from build123d import *

# Parameters (mm, degrees)
RESSALTO_EXTRUS_O1_DEPTH = 10.5
RESSALTO_EXTRUS_O2_START = -0.405481833
RESSALTO_EXTRUS_O2_DEPTH = 0.405481833
ESBO_O6_R                = 1.5
ESBO_O6_R_2              = 0.439880444
ESBO_O6_R_3              = 0.420000653
CORTE_EXTRUS_O1_DEPTH    = 10
ESBO_O7_R                = 2
CORTE_EXTRUS_O2_DEPTH    = 10
ESBO_O8_W                = 16.345048289
ESBO_O8_H                = 10.10072272
CORTE_EXTRUS_O3_DEPTH    = 6


with BuildPart() as part:
    # Esboço1 → Ressalto-extrusão1 (new body)
    with BuildSketch(Plane.XZ.offset(-2000)):
        with BuildLine():
            Line((26.191736717, -104.725419486), (63.230487022, -104.725419486))
            ThreePointArc((63.230487022, -104.725419486), (64.096864483, -104.922813013), (64.79222464, -105.476029391))
            Line((64.79222464, -105.476029391), (75.753474335, -119.17759151))
            ThreePointArc((75.753474335, -119.17759151), (76.078993355, -119.764967722), (76.191736717, -120.426981605))
            Line((76.191736717, -120.426981605), (76.191736717, -135.371353563))
            ThreePointArc((76.191736717, -135.371353563), (75.847871178, -136.492611182), (74.934518069, -137.228306945))
            Line((74.934518069, -137.228306945), (56.549353262, -144.582372868))
            ThreePointArc((56.549353262, -144.582372868), (56.184786952, -144.689332259), (55.806571909, -144.725419486))
            Line((55.806571909, -144.725419486), (49.020163841, -144.725419486))
            Line((49.020163841, -144.725419486), (48.505389373, -144.65803617))
            Line((48.505389373, -144.65803617), (48.017411303, -144.455878196))
            Line((48.017411303, -144.455878196), (47.605950279, -144.139633048))
            Line((47.605950279, -144.139633048), (46.777523154, -143.311205924))
            ThreePointArc((46.777523154, -143.311205924), (46.128676457, -142.877660421), (45.363309592, -142.725419486))
            Line((45.363309592, -142.725419486), (26.191736717, -142.725419486))
            Line((26.191736717, -142.725419486), (26.191736717, -104.725419486))
        make_face()
        with BuildLine():
            Line((48.266993092, -143.386462299), (47.484629935, -142.604099142))
            ThreePointArc((47.484629935, -142.604099142), (46.511359889, -141.953780888), (45.363309592, -141.725419486))
            Line((45.363309592, -141.725419486), (27.191736717, -141.725419486))
            Line((27.191736717, -141.725419486), (27.191736717, -105.725419486))
            Line((27.191736717, -105.725419486), (63.230487022, -105.725419486))
            ThreePointArc((63.230487022, -105.725419486), (63.663675752, -105.82411625), (64.011355831, -106.100724438))
            Line((64.011355831, -106.100724438), (74.972605526, -119.802286557))
            ThreePointArc((74.972605526, -119.802286557), (75.135365036, -120.095974663), (75.191736717, -120.426981605))
            Line((75.191736717, -120.426981605), (75.191736717, -135.371353563))
            ThreePointArc((75.191736717, -135.371353563), (75.019803947, -135.931982372), (74.563127393, -136.299830254))
            Line((74.563127393, -136.299830254), (56.177962586, -143.653896177))
            ThreePointArc((56.177962586, -143.653896177), (55.995679431, -143.707375873), (55.806571909, -143.725419486))
            Line((55.806571909, -143.725419486), (49.085335215, -143.725419486))
            Line((49.085335215, -143.725419486), (48.766120713, -143.683634718))
            Line((48.766120713, -143.683634718), (48.522121146, -143.582551368))
            Line((48.522121146, -143.582551368), (48.266993092, -143.386462299))
        make_face(mode=Mode.SUBTRACT)
    extrude(amount=RESSALTO_EXTRUS_O1_DEPTH)

    # Esboço5 → Ressalto-extrusão2 (add)
    with BuildSketch(Plane.XZ.offset(-1989.5).offset(RESSALTO_EXTRUS_O2_START)):
        with BuildLine():
            Line((27.191736717, -105.725419486), (63.230487022, -105.725419486))
            ThreePointArc((63.230487022, -105.725419486), (63.663675752, -105.82411625), (64.011355831, -106.100724438))
            Line((64.011355831, -106.100724438), (74.972605526, -119.802286557))
            ThreePointArc((74.972605526, -119.802286557), (75.135365036, -120.095974663), (75.191736717, -120.426981605))
            Line((75.191736717, -120.426981605), (75.191736717, -135.371353563))
            ThreePointArc((75.191736717, -135.371353563), (75.019803947, -135.931982372), (74.563127393, -136.299830254))
            Line((74.563127393, -136.299830254), (56.177962586, -143.653896177))
            ThreePointArc((56.177962586, -143.653896177), (55.995679431, -143.707375873), (55.806571909, -143.725419486))
            Line((55.806571909, -143.725419486), (49.085335215, -143.725419486))
            ThreePointArc((49.085335215, -143.725419486), (48.642453796, -143.637327588), (48.266993092, -143.386462299))
            Line((48.266993092, -143.386462299), (47.484629935, -142.604099142))
            ThreePointArc((47.484629935, -142.604099142), (46.511359889, -141.953780888), (45.363309592, -141.725419486))
            Line((45.363309592, -141.725419486), (27.191736717, -141.725419486))
            Line((27.191736717, -141.725419486), (27.191736717, -105.725419486))
        make_face()
    extrude(amount=RESSALTO_EXTRUS_O2_DEPTH)

    # Esboço6 → Corte-extrusão1 (cut)
    with BuildSketch(Plane.XZ.offset(-1989.5)):
        with Locations(Location((51.191736717, -118.225419486, 0), (0, 0, 270))):
            Circle(ESBO_O6_R)
        with Locations(Location((51.191736717, -133.225419486, 0), (0, 0, 270))):
            Circle(ESBO_O6_R)
        with Locations(Location((72.191736717, -130.725419486, 0), (0, 0, 270))):
            Circle(ESBO_O6_R)
        with Locations(Location((53.191736717, -139.725419486, 0), (0, 0, 270))):
            Circle(ESBO_O6_R)
        with Locations(Location((28.899554792, -108.599940214, 0), (0, 0, 270))):
            Circle(ESBO_O6_R_2)
        with Locations(Location((29.339435236, -139.725419486, 0), (0, 0, 270))):
            Circle(ESBO_O6_R_3)
    extrude(amount=-CORTE_EXTRUS_O1_DEPTH, mode=Mode.SUBTRACT)

    # Esboço7 → Corte-extrusão2 (cut)
    with BuildSketch(Plane.ZY.offset(-26.191736717)):
        with Locations(Location((-137.725419486, 1995.5, 0), (0, 0, 270))):
            Circle(ESBO_O7_R)
        with Locations(Location((-109.725419486, 1995.5, 0), (0, 0, 270))):
            Circle(ESBO_O7_R)
    extrude(amount=-CORTE_EXTRUS_O2_DEPTH, mode=Mode.SUBTRACT)

    # Esboço8 → Corte-extrusão3 (cut)
    with BuildSketch(Plane(origin=(0, 0, -144.725419486), x_dir=(-1, 0, 0), z_dir=(0, 0, -1))):
        with Locations((-46.726167809, 1994.995129696)):
            Rectangle(ESBO_O8_W, ESBO_O8_H)
    extrude(amount=-CORTE_EXTRUS_O3_DEPTH, mode=Mode.SUBTRACT)


solid = part.part
Work out the finished part from the listing and answer in its coordinate system (mm). A direction names the side the tool comes from. Round coordinates to 2 decimals unless told otherwise and drop trailing zeros. Order: outer loops, then holes, each group sorted by start corner. A loop starts at its lowest first (then second) coordinate and runs counter-clockwise, first axis right, second up. Notation, with made-up numbers: M 71,45 L 95,45 A16 cw 95,51 Z; hole C 73.5,80 d11. An arc over 180 degrees is marked long. Put each result on its own line as item: value. Start each with the question number.
Q1. Section A-A, the plane y = 1995.5 is taken. Give the number of separate pieces and of enclosed holes in the cut face, and give its area (3 significant figures).
Q2. Section B-B, the plane y = 1990.75 is taken. Write down the section's boundary in (x, z), and give its area (3 significant figures).
Q3. Section C-C, the plane z = -123 is taken. Write down the section's boundary in (x, y).
Q4. Flat-ended cylindrical pins translate along their axes: pin 1 (1.1 mm diameter, centred on y = 1994.5, z = -144, fed in from -X); pin 2 (3 mm diameter, centred on x = 52.5, y = 1994, fed in from -Z); pin 3 (5 mm diameter, centred on y = 1996, z = -115.5, fed in from +X); pin 4 (6 mm diameter, centred on x = 58, y = 1996, fed in from -Z). Find the tip coordinate at first contact, or state that the pin passes through.
Q5. Section D-D, the plane x = 33 is taken. Write down the section's boundary in (y, z).
Q6. Straight lines are drawn through the part: L1, parallel to Z at x = 26.6, y = 1995.5; L2, parallel to Z at x = 35, y = 1990.5; L3, parallel to X at y = 1998.75, z = -121.5. For each, find the intervals that lie inside material, in ascending order. Write a range as [from, to].
Q7. A tool of negligible diameter and unlimited length cuts with its end or side. For faces 4 (the flat face through (34, 1995, -142.725)), 5 (the flat face through (27.192, 1995, -124)), 6 (the flat face through (44, 1995, -104.725)), 7 (the cylindrical face through (26.7, 1993.6, -137.1)), 8 (the flat face through (47, 1989.945, -143)), from which of +Z, -Z, +X, -X, +Y, -Y can it reach the whole face along a straight path? Write none if from no direction.
Q8. For a pull along X with two mould halves and no side action, classify faces 1 (the flat face through (54.899, 1995, -144)), 2 (the cylindrical face through (72.258, 1989.7, -129.227)), 3 (the cylindrical face through (64.09, 1994.82, -104.92)) as pulls with the +X half, pulls with the -X half, needs draft (parallel to the pull), parting line crosses it, or undercut.
Findings below:
1. separate pieces: 3
1. enclosed holes: 0
1. area: 135 mm^2
2. outline: M 26.19,-142.73 L 38.55,-142.73 L 38.55,-141.73 L 27.19,-141.73 L 27.19,-105.73 L 63.23,-105.73 A1 cw 64.01,-106.1 L 74.97,-119.8 A1 cw 75.19,-120.43 L 75.19,-135.37 A1 cw 74.56,-136.3 L 56.18,-143.65 A1 cw 55.81,-143.73 L 54.9,-143.73 L 54.9,-144.73 L 55.81,-144.73 A2 ccw 56.55,-144.58 L 74.93,-137.23 A2 ccw 76.19,-135.37 L 76.19,-120.43 A2 ccw 75.75,-119.18 L 64.79,-105.48 A2 ccw 63.23,-104.73 L 26.19,-104.73 Z
2. area: 143 mm^2
3. outline: M 26.19,1989.5 L 76.19,1989.5 L 76.19,2000 L 75.19,2000 L 75.19,1989.91 L 27.19,1989.91 L 27.19,2000 L 26.19,2000 Z
4. pin 1: stops at x = 54.9
4. pin 2: stops at z = -105.73
4. pin 3: stops at x = 74.81
4. pin 4: stops at z = -144.73
5. outline: M 1989.5,-142.73 L 2000,-142.73 L 2000,-141.73 L 1989.91,-141.73 L 1989.91,-105.73 L 2000,-105.73 L 2000,-104.73 L 1989.5,-104.73 Z
6. L1: z = [-142.73, -139.73], [-135.73, -111.73], [-107.73, -104.73]
6. L2: z = [-142.73, -141.73], [-105.73, -104.73]
6. L3: x = [26.19, 27.19], [75.19, 76.19]
7. face 4: -Z, -X, +Y, -Y
7. face 5: +Y
7. face 6: +Z, +X, -X, +Y, -Y
7. face 7: -X
7. face 8: -Z, +Y
8. face 1: pulls with the -X half
8. face 2: undercut
8. face 3: pulls with the +X half
